```python
from build123d import *

# Parameters (mm, degrees)
F1_DEPTH       = 40
F5_D           = 3.5
F5_DEPTH       = 20
F5_CSINK_D     = 6
F5_CSINK_ANGLE = 90
F5_TIP         = 1.0515060833
F7_D           = 3.5
F7_DEPTH       = 20
F7_CSINK_D     = 6
F7_CSINK_ANGLE = 90
F7_TIP         = 1.0515060833
F8_R           = 3
F9_R           = 1


with BuildPart() as f1:
    # F0 (on Top) → F1 (new body)
    with BuildSketch(Plane.XY):
        with BuildLine():
            ThreePointArc((-35.5, 0), (0, 35.5), (35.5, 0))
            Line((35.5, 0), (55, 0))
            ThreePointArc((55, 0), (0, 55), (-55, 0))
            Line((-55, 0), (-35.5, 0))
        make_face()
    extrude(amount=F1_DEPTH)

    # F2 (on face) → F3 (revolve, cut)
    with BuildSketch(Plane.XZ):
        Polygon((51, 20), (55, 20), (55, 23), (51, 21), align=None)
        Polygon((51, 19), (55, 17), (55, 20), (51, 20), align=None)
    revolve(axis=Axis((0, 0, 0), (0, 0, -1)), mode=Mode.SUBTRACT)

    # F5
    with Locations(Plane.XZ):
        with Locations((43.25, 20)):
            CounterSinkHole(F5_D / 2, F5_CSINK_D / 2, depth=F5_DEPTH, counter_sink_angle=F5_CSINK_ANGLE)
            with Locations((0, 0, -(F5_DEPTH + F5_TIP / 2))):  # 118° drill point
                Cone(0, F5_D / 2, F5_TIP, mode=Mode.SUBTRACT)

    # F7
    with Locations(Plane.XZ):
        with Locations((-43.25, 20)):
            CounterSinkHole(F7_D / 2, F7_CSINK_D / 2, depth=F7_DEPTH, counter_sink_angle=F7_CSINK_ANGLE)
            with Locations((0, 0, -(F7_DEPTH + F7_TIP / 2))):  # 118° drill point
                Cone(0, F7_D / 2, F7_TIP, mode=Mode.SUBTRACT)

    # F8
    f8_edges = [f1.edges().sort_by_distance(p)[0] for p in [
        (0, 55, 0),
        (0, 55, 40),
    ]]
    fillet(f8_edges, radius=F8_R)

    # F9
    f9_edges = [f1.edges().sort_by_distance(p)[0] for p in [
        (0, 55, 23),
        (0, 55, 17),
    ]]
    fillet(f9_edges, radius=F9_R)


solid = f1.part
```
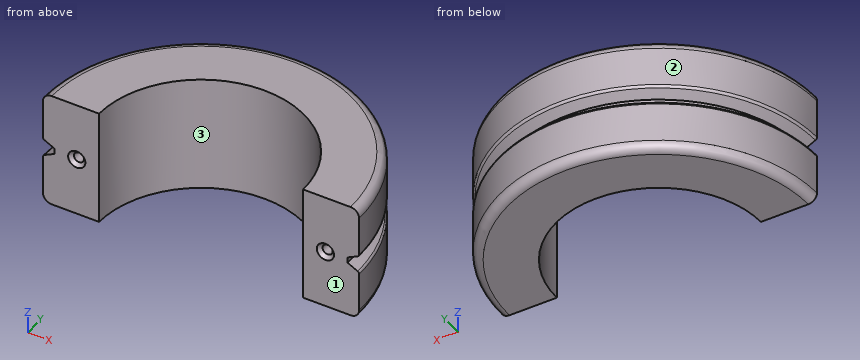
Input: part model. Units: mm. Frame: model coordinates. Face numbers are marked on the shaded views. Give positions to 0.01 mm unless a question says otherwise; leave off trailing zeros. Order: outer loops, then holes, each group sorted by start corner. A loop starts at its lowest first (then second) coordinate and runs counter-clockwise, first axis right, second up. Notation, with made-up numbers: M -2,-20 L 52,-20 A18 cw 52,6 Z; hole C 33,-36 d11. An arc over 180 degrees is marked long. Return JSON: item names as keys, results as strings.
Item 1: Cut plane B-B (y = 17.5). State how many separate pieces and enclosed holes the cut face has, then the cut area to 3 significant figures.
Solutions:
{"separate pieces": "2", "enclosed holes": "2", "area": "1,640 mm^2"}
Item 2: First-contact query: P1, Ø5, axis at x = -23.5, y = 30, coming from the -Z side; P2, Ø5, axis at y = 40, z = 8, coming from the +X side; P3, Ø3, axis at x = 4, z = 15.5, coming from the +Y side; P4, Ø3, axis at x = -28, y = 49.5, coming from the -Z side. Flat tips, straight axial feed; report the tip coordinate or a pass-through.
Solutions:
{"P1": "z = 0", "P2": "x = 40.23", "P3": "y = 54.94", "P4": "through"}
Item 3: Cut plane A-A (z = 35.5). Return loops of the section in (x, y).
Solutions:
{"outline": "M -55,0 L -35.5,0 A35.5 cw 35.5,0 L 55,0 A55 ccw Z"}
Item 4: Pull-direction query (X, two-part tool) for the marked faces 1, 2 and 3; classes: +X half, -X half, draft (parallel to the pull), parting line (faces both ways), or undercut.
Solutions:
{"face 1": "draft", "face 2": "parting line", "face 3": "undercut"}
Item 5: Ray query, probe 1 along X at (y, z) = (7, 20); probe 2 along X at (y, z) = (6, 20); probe 3 along Z at (x, y) = (-43, 8). Return the intervals inside material, ascending.
Solutions:
{"probe 1": "-50.52 to -45, -41.5 to -34.8, 34.8 to 41.5, 45 to 50.52", "probe 2": "-50.65 to -45, -41.5 to -34.99, 34.99 to 41.5, 45 to 50.65", "probe 3": "0 to 18.27, 21.73 to 40"}
